from build123d import *

# Parameters (mm, degrees)
SKETCH3_R           = 3.6
BOSS_EXTRUDE1_DEPTH = 7.2
SKETCH4_R           = 2.25
BOSS_EXTRUDE2_DEPTH = 2.5
BOSS_EXTRUDE3_START = 2.5
SKETCH5_R           = 2.25
BOSS_EXTRUDE3_DEPTH = 2.5
CHAMFER1_SIZE       = 0.5


with BuildPart() as part:
    # Sketch3 → Boss-Extrude1 (new body)
    with BuildSketch(Plane.XY):
        Circle(SKETCH3_R)
    extrude(amount=BOSS_EXTRUDE1_DEPTH)

    # Sketch4 → Boss-Extrude2 (add)
    with BuildSketch(Plane.XY):
        Circle(SKETCH4_R)
    extrude(amount=-BOSS_EXTRUDE2_DEPTH)

    # Sketch5 → Boss-Extrude3 (add)
    with BuildSketch(Plane.XY.offset(7.2).offset(BOSS_EXTRUDE3_START)):
        Circle(SKETCH5_R)
    extrude(amount=-BOSS_EXTRUDE3_DEPTH)

    # Chamfer1
    chamfer1_edges = [part.edges().sort_by_distance(p)[0] for p in [
        (-2.25, 0, -2.5),
    ]]
    chamfer(chamfer1_edges, length=CHAMFER1_SIZE)


solid = part.part
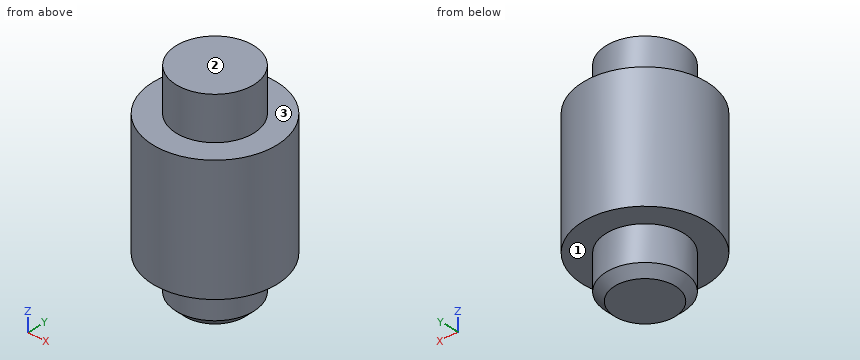
The listing builds one solid part. Answer for the finished solid, in the listing's coordinates (mm). Face numbers are marked on the shaded views. A direction names the side the tool comes from. Round coordinates to 2 decimals unless told otherwise and drop trailing zeros. Order: outer loops, then holes, each group sorted by start corner. A loop starts at its lowest first (then second) coordinate and runs counter-clockwise, first axis right, second up. Notation, with made-up numbers: M 79.5,31.25 L 138.5,31.25 A21 ccw 138.5,50.25 Z; hole C -12.75,57 d3. An arc over 180 degrees is marked long. Answer in a Markdown table with one row per item. Add a question column.
1) The part is cut by section C-C on y = 3.25. Determine the outline of the cut face in (x, z).
2) A flat-ended cylindrical pin translates along its axis: pin 1 Ø1.5 at (x, z) = (-1.5, 0) entering from +Y. Find the tip coordinate at first contact, or state that the pin passes through.
3) The part is cut by section B-B on z = 4.5. Determine the outline of the cut face in (x, y).
4) Consider line 1 along Z through (x, y) = (-2.75, 0.75); line 2 along Y through (x, z) = (2.75, 1.5); line 3 along Y through (x, z) = (-0.5, -1.5). Determine where each line is inside the solid, lowest interval first. Write a range as from..to.
5) The part is cut by section D-D on z = -1.5. Determine the outline of the cut face in (x, y), plus the area to 3 significant figures.
6) The part is cut by section A-A on x = 0. Determine the outline of the cut face in (y, z), plus the area to 3 significant figures.
7) Which of the six approach directions +Z, -Z, +X, -X, +Y, -Y give full straight-line access (tool end or side, diameter ignored) to the marked faces 1, 2 and 3?
Findings below:
| question | item | result |
|---|---|---|
| 1 | outline | M -1.55,0 L 1.55,0 L 1.55,7.2 L -1.55,7.2 Z |
| 2 | pin 1 | stops at y = 3.52 |
| 3 | outline | C 0,0 d7.2 |
| 4 | line 1 | z = 0..7.2 |
| 4 | line 2 | y = -2.32..2.32 |
| 4 | line 3 | y = -2.19..2.19 |
| 5 | outline | C 0,0 d4.5 |
| 5 | area | 15.9 mm² |
| 6 | outline | M -3.6,0 L -2.25,0 L -2.25,-2 L -1.75,-2.5 L 1.75,-2.5 L 2.25,-2 L 2.25,0 L 3.6,0 L 3.6,7.2 L 2.25,7.2 L 2.25,9.7 L -2.25,9.7 L -2.25,7.2 L -3.6,7.2 Z |
| 6 | area | 74.1 mm² |
| 7 | face 1 | -Z |
| 7 | face 2 | +Z, +X, -X, +Y, -Y |
| 7 | face 3 | +Z |
